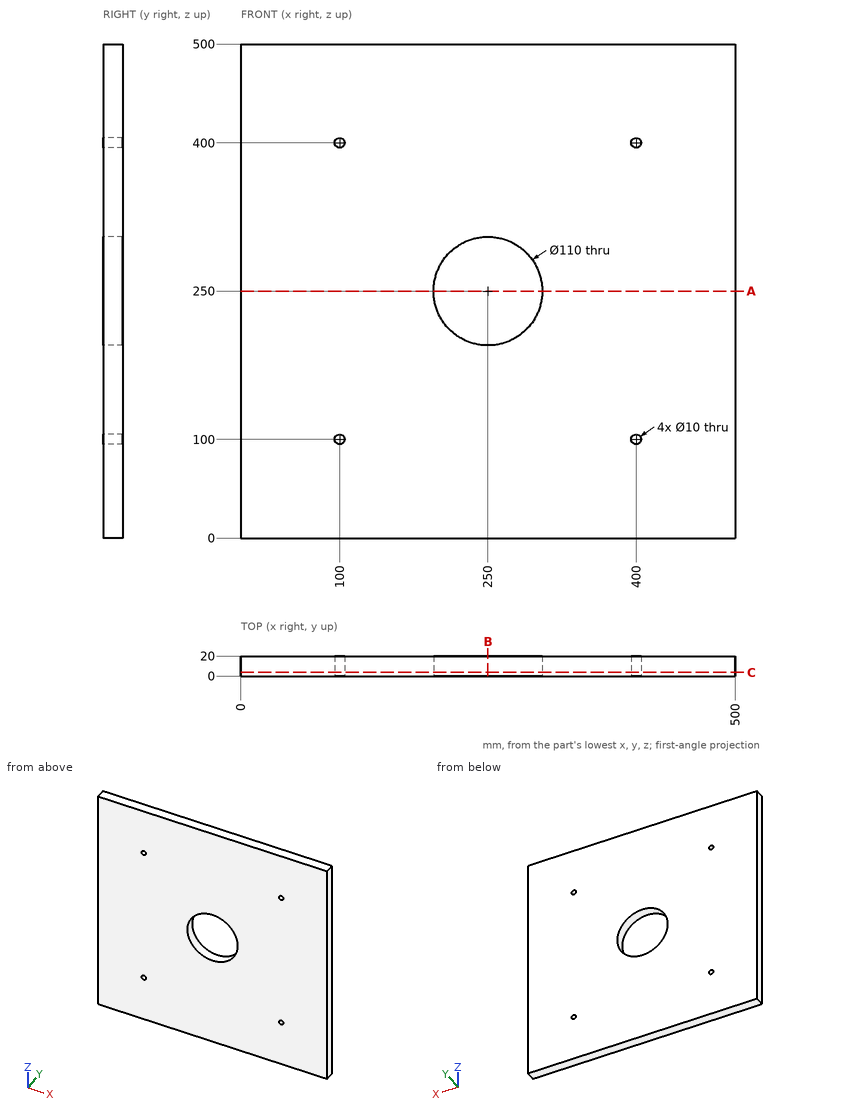
Input: dimensioned drawing with shaded views. Units: mm. Origin: part minimum x, y, z. Coordinates: 2 decimals unless noted, no trailing zeros. Loops run counter-clockwise (first coordinate to the right, second up) from the corner with the lowest first, then second, coordinate; pieces in that order, holes last. Notation, with made-up numbers: M -11,-29.5 L 11,-29.5 A18 cw 11,-24.5 Z; hole C 42,44.25 d5. An arc over 180 degrees is marked long. Use a Markdown table: item, result. Add a question column.
1) Line query: L1, parallel to Z at x = 400, y = 11.5; L2, parallel to X at y = 13.75, z = 205.5. Output: solid intervals per line, ascending. Write a range as from..to.
2) Section B-B, the plane x = 250. Return the cut outline in (y, z).
3) Section A-A, the plane z = 250. Return the cut outline in (x, y), plus the area to 3 significant figures.
4) Section C-C, the plane y = 3.75. Return the cut outline in (x, z).
Answer below:
| question | item | result |
|---|---|---|
| 1 | L1 | 0..95, 105..395, 405..500 |
| 1 | L2 | 0..217.68, 282.32..500 |
| 2 | outline | M 0,0 L 20,0 L 20,195 L 0,195 Z; M 0,305 L 20,305 L 20,500 L 0,500 Z |
| 3 | outline | M 0,0 L 195,0 L 195,20 L 0,20 Z; M 305,0 L 500,0 L 500,20 L 305,20 Z |
| 3 | area | 7,800 mm2 |
| 4 | outline | M 0,0 L 500,0 L 500,500 L 0,500 Z; hole C 100,100 d10; hole C 100,400 d10; hole C 250,250 d110; hole C 400,100 d10; hole C 400,400 d10 |
